The model under review builds one solid part; all positions refer to its coordinate system, in mm. A direction names the side the tool comes from. Round coordinates to 2 decimals unless told otherwise and drop trailing zeros. Write each loop counter-clockwise with the first axis right and the second up, starting at its lowest first coordinate (ties: lowest second). Pieces come first, ordered by that corner, then holes.
Item 1: Draft analysis for pull direction X (two halves, no side actions). For faces 3 (the face through (52, 0, 20)), 4 (the face through (60, -15, 15)), 5 (the face through (20, -18, 7)), 6 (the face through (44.93, -36.302, 5.07)), state which applies: +X half, -X half, draft (parallel to the pull), parting line (faces both ways), or undercut.
Item 2: Clearance check with flat-ended pins moving along their axes: pin 1 Ø6 at (x, y) = (28.5, -20) entering from +Z; pin 2 Ø6 at (x, y) = (7.5, -6) entering from +Z. State where each tip first meets the part, or that it passes through.
Item 3: Add section C-C (z = 29.5). Give the boundary of the cut face in (x, y), plus the area to 3 significant figures.
Item 4: Add section A-A (y = -20). Give the boundary of the cut face in (x, z).
Item 5: To check wall thickness, follow L1, parallel to X at y = -2, z = 9.5; L2, parallel to X at y = -8.5, z = 4.5; L3, parallel to X at y = -19, z = 23. State the ranges of each line that lie inside material, in increasing order.
Item 6: Machinability: for faces 1 (the face through (30, -20, 10)), 2 (the face through (8, -20, 25)), which of the approach directions +Z, -Z, +X, -X, +Y, -Y give a long, thin tool a straight path to every point of the face, cutting with its end or side? Answer none if there is none.
Item 7: Add section D-D (y = -37). Give the boundary of the cut face in (x, z), plus the area to 3 significant figures.
Item 8: Add section B-B (x = 17). Give the boundary of the cut face in (y, z).
```python
from build123d import *

# Parameters (mm, degrees)
F0_W     = 60
F0_H     = 40
F1_DEPTH = 40
F2_W     = 20
F2_H     = 30
F3_DEPTH = 40
F5_DEPTH = 60
F8_DEPTH = 40


# Not quite as in the source:
# - a feature of the source that left no trace in its solid (it failed there, or was rolled back) is left out


with BuildPart() as f1:
    # F0 (on Front) → F1 (new body)
    with BuildSketch(Plane.XZ):
        with Locations((30, 20)):
            Rectangle(F0_W, F0_H)
    extrude(amount=F1_DEPTH)

    # F2 (on face) → F3 (cut)
    with BuildSketch(Plane.XZ.offset(40)):
        with Locations((30, 25)):
            Rectangle(F2_W, F2_H)
    extrude(amount=-F3_DEPTH, mode=Mode.SUBTRACT)

    # F4 (on face) → F5 (cut)
    with BuildSketch(Plane.YZ.offset(60)):
        Polygon((-40, 40), (-40, 10), (0, 40), align=None)
    extrude(amount=-F5_DEPTH, mode=Mode.SUBTRACT)

    # F6 (on face) + F7 (on face) → F8 (cut)
    with BuildSketch(Plane(origin=(0, -19.2, 25.6), x_dir=(1, 0, 0), z_dir=(0, -0.6, 0.8))):
        Polygon((20, -26), (20, 24), (10, -26), align=None)
    with BuildSketch(Plane(origin=(0, -19.2, 25.6), x_dir=(1, 0, 0), z_dir=(0, -0.6, 0.8))):
        Polygon((50, -26), (40, 24), (40, -26), align=None)
    extrude(amount=-F8_DEPTH, mode=Mode.SUBTRACT)


solid = f1.part
```
Numbers:
1. face 3: draft
1. face 4: +X half
1. face 5: undercut
1. face 6: undercut
2. pin 1: stops at z = 10
2. pin 2: stops at z = 37.75
3. outline: (0, -14) - (16.5, -14) - (18.74, 0) - (0, 0) - close; (41.26, 0) - (43.5, -14) - (60, -14) - (60, 0) - close
3. area: 493 mm2
4. outline: (0, 0) - (12, 0) - (15, 25) - (0, 25) - close; (20, 0) - (40, 0) - (40, 10) - (20, 10) - close; (45, 25) - (48, 0) - (60, 0) - (60, 25) - close
5. L1: x = 0 to 16.02, 20 to 40, 43.98 to 60
5. L2: x = 0 to 14.38, 20 to 40, 45.62 to 60
5. L3: x = 0 to 14.92, 45.08 to 60
6. face 1: +Z, +Y, -Y
6. face 2: +Z, +X, -X, -Y
7. outline: (0, 0) - (60, 0) - (60, 12.25) - (49.25, 12.25) - (50, 6) - (40, 6) - (40, 10) - (20, 10) - (20, 6) - (10, 6) - (10.75, 12.25) - (0, 12.25) - close
7. area: 570 mm2
8. outline: (-40, 0) - (-32.5, 0) - (-40, 10) - close; (-12, 31) - (0, 15) - (0, 40) - close
